from build123d import *

# Parameters (mm, degrees)
SKETCH1_R           = 1.1684
SKETCH1_W           = 1.5
SKETCH1_H           = 33.75
BOSS_EXTRUDE1_DEPTH = 3.175


with BuildPart() as part:
    # Sketch1 → Boss-Extrude1 (new body)
    with BuildSketch(Plane.XY):
        with BuildLine():
            Line((-31.453240404, -3.582490692), (-31.453240404, -46.222490692))
            ThreePointArc((-31.453240404, -46.222490692), (-32.197189179, -48.018541916), (-33.993240404, -48.762490692))
            Line((-33.993240404, -48.762490692), (-44.383240404, -48.762490692))
            ThreePointArc((-44.383240404, -48.762490692), (-46.179291628, -48.018541916), (-46.923240404, -46.222490692))
            Line((-46.923240404, -46.222490692), (-46.923240404, -32.850740692))
            ThreePointArc((-46.923240404, -32.850740692), (-47.667189179, -31.054689467), (-49.463240404, -30.310740692))
            Line((-49.463240404, -30.310740692), (-51.065740404, -30.310740692))
            ThreePointArc((-51.065740404, -30.310740692), (-52.861791628, -29.566791916), (-53.605740404, -27.770740692))
            Line((-53.605740404, -27.770740692), (-53.605740404, -8.784240692))
            ThreePointArc((-53.605740404, -8.784240692), (-52.861791628, -6.988189467), (-51.065740404, -6.244240692))
            Line((-51.065740404, -6.244240692), (-49.463240404, -6.244240692))
            ThreePointArc((-49.463240404, -6.244240692), (-47.667189179, -5.500291916), (-46.923240404, -3.704240692))
            Line((-46.923240404, -3.704240692), (-46.923240404, -3.582490692))
            ThreePointArc((-46.923240404, -3.582490692), (-46.179291628, -1.786439467), (-44.383240404, -1.042490692))
            Line((-44.383240404, -1.042490692), (-33.993240404, -1.042490692))
            ThreePointArc((-33.993240404, -1.042490692), (-32.197189179, -1.786439467), (-31.453240404, -3.582490692))
        make_face()
        with Locations((-43.430740404, -4.534990692)):
            Circle(SKETCH1_R, mode=Mode.SUBTRACT)
        with Locations((-34.945740404, -4.534990692)):
            Circle(SKETCH1_R, mode=Mode.SUBTRACT)
        with Locations((-43.430740404, -45.269990692)):
            Circle(SKETCH1_R, mode=Mode.SUBTRACT)
        with Locations((-34.945740404, -45.269990692)):
            Circle(SKETCH1_R, mode=Mode.SUBTRACT)
        with Locations((-50.113240404, -9.736740692)):
            Circle(SKETCH1_R, mode=Mode.SUBTRACT)
        with Locations((-50.113240404, -26.818240692)):
            Circle(SKETCH1_R, mode=Mode.SUBTRACT)
        with Locations((-39.188240404, -24.902490692)):
            Rectangle(SKETCH1_W, SKETCH1_H, mode=Mode.SUBTRACT)
    extrude(amount=BOSS_EXTRUDE1_DEPTH)


solid = part.part
The listing builds one solid part. Answer for the finished solid, in the listing's coordinates (mm). A direction names the side the tool comes from. Give positions to 0.01 mm unless a question says otherwise; leave off trailing zeros. Loops run counter-clockwise (first coordinate to the right, second up) from the corner with the lowest first, then second, coordinate; pieces in that order, holes last. Notation, with made-up numbers: (26, -9.5) - (85, -9.5) arc R25 ccw to (85, 6.5) - close; hole circle Ø9 at (53, 66.5). An arc over 180 degrees is marked (long way). Use one line per item in the form item = value.
1. Find the intervals of material crossed by line 1 along Y through (x, z) = (-43.5, 1.2); line 2 along Y through (x, z) = (-39.5, 0.6); line 3 along X through (y, z) = (-21, 0.7), in increasing order. Write a range as [from, to].
Calculated:
line_1 = [-48.76, -46.44], [-44.1, -5.7], [-3.37, -1.04]
line_2 = [-48.76, -41.78], [-8.03, -1.04]
line_3 = [-53.61, -39.94], [-38.44, -31.45]
2. The mould has two halves that part along X. Classify faces 1 (the face through (-39.938, -25, 2)), 2 (the face through (-46.2, -1.81, 1.57)), 3 (the face through (-50, -30.311, 2)), 4 (the face through (-38.438, -25, 2)): pulls with the +X half, pulls with the -X half, needs draft (parallel to the pull), parting line crosses it, or undercut.
Calculated:
face_1 = undercut
face_2 = pulls with the -X half
face_3 = needs draft
face_4 = undercut
3. Given pin 1 Ø1 at (x, y) = (-40, -24.5) entering from -Z; pin 2 Ø1.3 at (x, z) = (-50.5, 1) entering from -Y; pin 3 Ø1.3 at (x, z) = (-50.5, 2) entering from +Y, each flat-ended and moving along its own axis, determine where each tip first touches the part or whether it passes through.
Calculated:
pin_1 = 0
pin_2 = -30.31
pin_3 = -6.24
4. Section D-D on y = -14 is taken. Give the vertices of the cut face in (x, z) (3 decimals).
Calculated:
outline = (-53.606, 0) - (-39.938, 0) - (-39.938, 3.175) - (-53.606, 3.175) - close; (-38.438, 0) - (-31.453, 0) - (-31.453, 3.175) - (-38.438, 3.175) - close
5. Section C-C on y = -5 is taken. Give the vertices of the cut face in (x, z) (3 decimals).
Calculated:
outline = (-47.279, 0) - (-44.503, 0) - (-44.503, 3.175) - (-47.279, 3.175) - close; (-42.359, 0) - (-36.018, 0) - (-36.018, 3.175) - (-42.359, 3.175) - close; (-33.874, 0) - (-31.453, 0) - (-31.453, 3.175) - (-33.874, 3.175) - close
6. Section B-B on x = -50.5 is taken. Give the vertices of the cut face in (y, z) (3 decimals).
Calculated:
outline = (-30.311, 0) - (-27.921, 0) - (-27.921, 3.175) - (-30.311, 3.175) - close; (-25.716, 0) - (-10.839, 0) - (-10.839, 3.175) - (-25.716, 3.175) - close; (-8.634, 0) - (-6.244, 0) - (-6.244, 3.175) - (-8.634, 3.175) - close
7. Which of the six approach directions +Z, -Z, +X, -X, +Y, -Y give full straight-line access (tool end or side, diameter ignored) to faces 5 (the face through (-46.923, -40, 2)), 6 (the face through (-39, -41.777, 2)), 7 (the face through (-53.606, -18, 2))?
Calculated:
face_5 = +Z, -Z, -X, -Y
face_6 = +Z, -Z
face_7 = +Z, -Z, -X, +Y, -Y
8. Section A-A on y = -35 is taken. Give the vertices of the cut face in (x, z) (3 decimals).
Calculated:
outline = (-46.923, 0) - (-39.938, 0) - (-39.938, 3.175) - (-46.923, 3.175) - close; (-38.438, 0) - (-31.453, 0) - (-31.453, 3.175) - (-38.438, 3.175) - close
